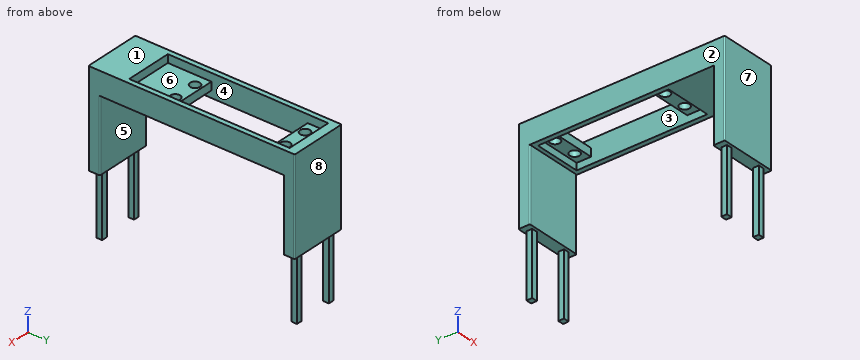
from build123d import *

# Parameters (mm, degrees)
BOSS_EXTRUDE1_OUTLINE_W   = 25
BOSS_EXTRUDE1_OUTLINE_H   = 5
BOSS_EXTRUDE1_OUTLINE_W_2 = 3
BOSS_EXTRUDE1_OUTLINE_H_2 = 3
BOSS_EXTRUDE1_DEPTH       = 31.595565731
SKETCH4_W                 = 25
SKETCH4_H                 = 90
BOSS_EXTRUDE3_DEPTH       = 10
SKETCH6_R                 = 2.15
CUT_EXTRUDE2_DEPTH        = 10
SKETCH7_W                 = 20.6
SKETCH7_H                 = 42
CUT_EXTRUDE3_DEPTH        = 10
SKETCH9_W                 = 2
SKETCH9_H                 = 90
CUT_EXTRUDE4_DEPTH        = 105.890618955
SKETCH10_W                = 2
SKETCH10_H                = 90
BOSS_EXTRUDE4_DEPTH       = 25
SKETCH8_W                 = 2.5
SKETCH8_H                 = 2.5
BOSS_EXTRUDE5_DEPTH       = 27.5
SKETCH11_W                = 3
SKETCH11_H                = 80
CUT_EXTRUDE5_DEPTH        = 123.742049491
SKETCH13_W                = 20.6
SKETCH13_H                = 57
CUT_EXTRUDE6_DEPTH        = 3
FILLET1_R                 = 0.5
SKETCH14_W                = 20.6
SKETCH14_H                = 70
CUT_EXTRUDE7_DEPTH        = 3.5


# Read off the part's stored shape, not the designer's step: Boss-Extrude1
with BuildPart() as part:
    # Boss-Extrude1 outline → Boss-Extrude1 (new body)
    # profile 1 of 2: a face of its own
    with BuildSketch(Plane.XY.offset(-60.133068515)):
        with Locations((125.570893714, 79.725640866)):
            Rectangle(BOSS_EXTRUDE1_OUTLINE_W, BOSS_EXTRUDE1_OUTLINE_H)
        with Locations((117.070893714, 79.725640866)):
            Rectangle(BOSS_EXTRUDE1_OUTLINE_W_2, BOSS_EXTRUDE1_OUTLINE_H_2, mode=Mode.SUBTRACT)
        with Locations((134.070893714, 79.725640866)):
            Rectangle(BOSS_EXTRUDE1_OUTLINE_W_2, BOSS_EXTRUDE1_OUTLINE_H_2, mode=Mode.SUBTRACT)
    # profile 2 of 2: a face of its own
    with BuildSketch(Plane.XY.offset(-60.133068515)):
        with Locations((125.570893714, -5.274359134)):
            Rectangle(BOSS_EXTRUDE1_OUTLINE_W, BOSS_EXTRUDE1_OUTLINE_H)
        with Locations((117.070893714, -5.274359134)):
            Rectangle(BOSS_EXTRUDE1_OUTLINE_W_2, BOSS_EXTRUDE1_OUTLINE_H_2, mode=Mode.SUBTRACT)
        with Locations((134.070893714, -5.274359134)):
            Rectangle(BOSS_EXTRUDE1_OUTLINE_W_2, BOSS_EXTRUDE1_OUTLINE_H_2, mode=Mode.SUBTRACT)
    extrude(amount=BOSS_EXTRUDE1_DEPTH)

    # Sketch4 → Boss-Extrude3 (add)
    with BuildSketch(Plane.XY.offset(-28.537502783)):
        with Locations((125.570893714, 37.225640866)):
            Rectangle(SKETCH4_W, SKETCH4_H)
    extrude(amount=BOSS_EXTRUDE3_DEPTH)

    # Sketch6 → Cut-Extrude2 (cut)
    with BuildSketch(Plane.XY.offset(-18.537502783)):
        with Locations((130.820893714, 24.225640866)):
            Circle(SKETCH6_R)
        with Locations((120.320893714, 24.225640866)):
            Circle(SKETCH6_R)
        with Locations((130.820893714, 72.225640866)):
            Circle(SKETCH6_R)
        with Locations((120.320893714, 72.225640866)):
            Circle(SKETCH6_R)
        with Locations((130.820893714, 72.225640866)):
            Circle(SKETCH6_R)
    extrude(amount=-CUT_EXTRUDE2_DEPTH, mode=Mode.SUBTRACT)

    # Sketch7 → Cut-Extrude3 (cut)
    with BuildSketch(Plane.XY.offset(-18.537502783)):
        with Locations((125.570893714, 48.225640866)):
            Rectangle(SKETCH7_W, SKETCH7_H)
    extrude(amount=-CUT_EXTRUDE3_DEPTH, mode=Mode.SUBTRACT)

    # Sketch9 → Cut-Extrude4 (cut, through all)
    with BuildSketch(Plane(origin=(138.070893714, 0, 0), x_dir=(0, 0, -1), z_dir=(1, 0, 0))):
        with Locations((59.133068515, 37.225640866)):
            Rectangle(SKETCH9_W, SKETCH9_H)
    extrude(amount=-CUT_EXTRUDE4_DEPTH, mode=Mode.SUBTRACT)

    # Sketch10 → Boss-Extrude4 (add)
    with BuildSketch(Plane(origin=(138.070893714, 0, 0), x_dir=(0, 0, -1), z_dir=(1, 0, 0))):
        with Locations((59.133068515, 37.225640866)):
            Rectangle(SKETCH10_W, SKETCH10_H)
    extrude(amount=-BOSS_EXTRUDE4_DEPTH)

    # Sketch8 → Boss-Extrude5 (add)
    with BuildSketch(Plane(origin=(0, 0, -60.133068515), x_dir=(-1, 0, 0), z_dir=(0, 0, -1))):
        Polygon((-135.320893714, 80.975640866), (-135.320893714, 78.475640866), (-132.820893714, 78.475640866), align=None)
        Polygon((-132.820893714, 80.975640866), (-132.820893714, 78.475640866), (-135.320893714, 80.975640866), align=None)
        Polygon((-118.320893714, 80.975640866), (-118.320893714, 78.475640866), (-115.820893714, 80.975640866), align=None)
        Polygon((-118.320893714, 78.475640866), (-115.820893714, 80.975640866), (-115.820893714, 78.475640866), align=None)
        with Locations((-117.070893714, -5.274359134)):
            Rectangle(SKETCH8_W, SKETCH8_H)
        with Locations((-134.070893714, -5.274359134)):
            Rectangle(SKETCH8_W, SKETCH8_H)
    extrude(amount=BOSS_EXTRUDE5_DEPTH)

    # Sketch11 → Cut-Extrude5 (cut, through all)
    with BuildSketch(Plane(origin=(138.070893714, 0, 0), x_dir=(0, 0, -1), z_dir=(1, 0, 0))):
        with Locations((59.633068515, 37.225640866)):
            Rectangle(SKETCH11_W, SKETCH11_H)
    extrude(amount=-CUT_EXTRUDE5_DEPTH, mode=Mode.SUBTRACT)

    # Sketch13 → Cut-Extrude6 (cut)
    with BuildSketch(Plane(origin=(0, 0, -28.537502783), x_dir=(-1, 0, 0), z_dir=(0, 0, -1))):
        with Locations((-125.570893714, 46.975640866)):
            Rectangle(SKETCH13_W, SKETCH13_H)
    extrude(amount=-CUT_EXTRUDE6_DEPTH, mode=Mode.SUBTRACT)

    # Fillet1
    fillet1_edges = [part.edges().sort_by_distance(p)[0] for p in [
        (113.070893714, -7.774359134, -38.335285649),
        (138.070893714, -7.774359134, -43.335285649),
        (138.070893714, 77.225640866, -43.335285649),
        (138.070893714, 82.225640866, -39.335285649),
        (113.070893714, 82.225640866, -43.335285649),
        (138.070893714, -2.774359134, -43.335285649),
        (113.070893714, 77.225640866, -43.335285649),
        (113.070893714, -2.774359134, -43.335285649),
    ]]
    fillet(fillet1_edges, radius=FILLET1_R)

    # Sketch14 → Cut-Extrude7 (cut)
    with BuildSketch(Plane.XY.offset(-18.537502783)):
        with Locations((125.570893714, 43.225640866)):
            Rectangle(SKETCH14_W, SKETCH14_H)
    extrude(amount=-CUT_EXTRUDE7_DEPTH, mode=Mode.SUBTRACT)


solid = part.part
Model file for the job. Use its own axes, mm. Face numbers are marked on the shaded views. A direction names the side the tool comes from. Give positions to 0.01 mm unless a question says otherwise; leave off trailing zeros. Loops run counter-clockwise (first coordinate to the right, second up) from the corner with the lowest first, then second, coordinate; pieces in that order, holes last.
1) Saw through at A-A (z = -42.5). Count the separate pieces of the cut face and the enclosed holes in it, plus the area to 3 significant figures.
2) Saw through at D-D (y = 57.5). Write the cut outline in (x, z).
3) Saw through at C-C (z = -82). Write the cut outline in (x, y), plus the area to 3 significant figures.
4) Wall check: line 1 (Y direction, x = 116.5, z = -54.5); line 2 (Y direction, x = 129.5, z = -29); line 3 (X direction, y = 30, z = -22). Give the ranges that are in metal, low to high.
5) Tool access for the marked faces 4, 5, 6, 7 and 8: list every direction of +Z, -Z, +X, -X, +Y, -Y with a clear straight run to the whole face (end or side of a thin tool).
6) Flat gauge pins, fed straight in: pin 1 Ø2 at (y, z) = (80, -74) entering from +X; pin 2 Ø8 at (x, z) = (132, -70.5) entering from +Y; pin 3 Ø2.5 at (x, y) = (128, -5) entering from -Z. Where does each tip first touch, or does it go through?
7) Pull direction X, two halves, no side cores. Call the marked faces 1, 2 and 3: +X half, -X half, draft (parallel to the pull), parting line (faces both ways), or undercut.
8) Saw through at B-B (x = 126.5). Write the cut outline in (y, z), plus the area to 3 significant figures.
Answer block:
1. separate pieces: 2
1. enclosed holes: 4
1. area: 214 mm2
2. outline: (113.07, -28.54) - (115.27, -28.54) - (115.27, -18.54) - (113.07, -18.54) - close; (135.87, -28.54) - (138.07, -28.54) - (138.07, -18.54) - (135.87, -18.54) - close
3. outline: (115.82, -6.52) - (118.32, -6.52) - (118.32, -4.02) - (115.82, -4.02) - close; (115.82, 78.48) - (118.32, 78.48) - (118.32, 80.98) - (115.82, 80.98) - close; (132.82, -6.52) - (135.32, -6.52) - (135.32, -4.02) - (132.82, -4.02) - close; (132.82, 78.48) - (135.32, 78.48) - (135.32, 80.98) - (132.82, 80.98) - close
3. area: 25.0 mm2
4. line 1: y = -7.77 to -6.77, -3.77 to -2.77, 77.23 to 78.23, 81.23 to 82.23
4. line 2: y = -7.77 to -2.77, 77.23 to 82.23
4. line 3: x = 113.07 to 115.27, 135.87 to 138.07
5. face 4: none
5. face 5: -Z, +X, -X
5. face 6: +Z
5. face 7: +Z, -Z, +X, -X, -Y
5. face 8: +Z, -Z, +X, -X, +Y
6. pin 1: stops at x = 135.32
6. pin 2: stops at y = 80.98
6. pin 3: stops at z = -60.13
7. face 1: draft
7. face 2: -X half
7. face 3: undercut
8. outline: (-7.77, -60.13) - (-2.77, -60.13) - (-2.77, -28.54) - (18.48, -28.54) - (18.48, -25.54) - (27.23, -25.54) - (27.23, -22.04) - (8.23, -22.04) - (8.23, -18.54) - (-7.77, -18.54) - close; (69.23, -25.54) - (75.48, -25.54) - (75.48, -28.54) - (77.23, -28.54) - (77.23, -60.13) - (82.23, -60.13) - (82.23, -18.54) - (78.23, -18.54) - (78.23, -22.04) - (69.23, -22.04) - close
8. area: 653 mm2
